Input: part model. Units: mm. Frame: model coordinates. A direction names the side the tool comes from. Coordinates: 2 decimals unless noted, no trailing zeros. Order: outer loops, then holes, each group sorted by start corner. A loop starts at its lowest first (then second) coordinate and runs counter-clockwise, first axis right, second up. Notation, with made-up numbers: M 68.25,22.5 L 80.25,22.5 A14 ccw 80.25,26.5 Z; hole C -31,74.25 d1. An arc over 180 degrees is marked long. Answer in a Markdown table with one row per item.
from build123d import *

# Parameters (mm, degrees)
SKETCH1_W                      = 41.4
SKETCH1_H                      = 33.02
SKETCH1_R                      = 3.175
BOSS_EXTRUDE1_DEPTH            = 12
SKETCH2_W                      = 41.4
SKETCH2_H                      = 6.51
BOSS_EXTRUDE2_DEPTH            = 53
CUT_EXTRUDE1_REACH             = 72.186
SKETCH4_R                      = 3.175
CUT_EXTRUDE1_DIRECTION_2_REACH = 72.186
CUT_EXTRUDE3_REACH             = 72.186
CUT_EXTRUDE3_DIRECTION_2_REACH = 72.186
CUT_EXTRUDE4_DEPTH             = 12
BOSS_EXTRUDE3_DEPTH            = 12
FILLET3_R                      = 3


with BuildPart() as part:
    # Sketch1 → Boss-Extrude1 (new body)
    with BuildSketch(Plane.XY):
        Rectangle(SKETCH1_W, SKETCH1_H)
        with Locations((12.7, 0)):
            Circle(SKETCH1_R, mode=Mode.SUBTRACT)
        with Locations((-12.7, 0)):
            Circle(SKETCH1_R, mode=Mode.SUBTRACT)
    extrude(amount=BOSS_EXTRUDE1_DEPTH)

    # Sketch2 → Boss-Extrude2 (add)
    with BuildSketch(Plane.XY.offset(12)):
        with Locations((0, 13.255)):
            Rectangle(SKETCH2_W, SKETCH2_H)
        with Locations((0, -13.255)):
            Rectangle(SKETCH2_W, SKETCH2_H)
    extrude(amount=BOSS_EXTRUDE2_DEPTH)

    # Cut-Extrude1: up to this face of the body (flat: up to its plane)
    cut_extrude1_end = Plane(part.part.faces().sort_by_distance((0, -16.51, 32.5))[0])
    # Sketch4 → Cut-Extrude1 (cut, up to the picked face)
    with BuildSketch(Plane(origin=(0, 0, 0), x_dir=(1, 0, 0), z_dir=(0, 1, 0)), mode=Mode.PRIVATE) as cut_extrude1_sk1:
        with Locations(Location((0, -35.5, 0), (0, 0, 270))):
            Circle(SKETCH4_R)
    cut_extrude1_tool1 = split(extrude(cut_extrude1_sk1.sketch, amount=-CUT_EXTRUDE1_REACH, mode=Mode.PRIVATE), bisect_by=cut_extrude1_end, keep=Keep.BOTH, mode=Mode.PRIVATE)
    add(cut_extrude1_tool1.solids().sort_by(Axis((0, 0, 35.5), (0, -1, 0)))[0], mode=Mode.SUBTRACT)

    # Cut-Extrude1 direction 2: up to this face of the body (flat: up to its plane)
    cut_extrude1_direction_2_end = Plane(part.part.faces().sort_by_distance((0, 16.51, 32.5))[0])
    # Sketch4 → Cut-Extrude1 direction 2 (cut, up to the picked face)
    with BuildSketch(Plane(origin=(0, 0, 0), x_dir=(1, 0, 0), z_dir=(0, 1, 0)), mode=Mode.PRIVATE) as cut_extrude1_direction_2_sk1:
        with Locations(Location((0, -35.5, 0), (0, 0, 270))):
            Circle(SKETCH4_R)
    cut_extrude1_direction_2_tool1 = split(extrude(cut_extrude1_direction_2_sk1.sketch, amount=CUT_EXTRUDE1_DIRECTION_2_REACH, mode=Mode.PRIVATE), bisect_by=cut_extrude1_direction_2_end, keep=Keep.BOTH, mode=Mode.PRIVATE)
    add(cut_extrude1_direction_2_tool1.solids().sort_by(Axis((0, 0, 35.5), (0, 1, 0)))[0], mode=Mode.SUBTRACT)

    # Cut-Extrude3: up to this face of the body (flat: up to its plane)
    cut_extrude3_end = Plane(part.part.faces().sort_by_distance((-19.929353518, -16.51, 32.5))[0])
    # Sketch6 → Cut-Extrude3 (cut, up to the picked face)
    with BuildSketch(Plane(origin=(0, 0, 0), x_dir=(1, 0, 0), z_dir=(0, 1, 0)), mode=Mode.PRIVATE) as cut_extrude3_sk1:
        with BuildLine():
            Line((-8, -35.5), (-8, -20))
            Line((-8, -20), (-8, -12))
            Line((-8, -12), (-16, -12))
            Line((-16, -12), (-20.7, -12))
            Line((-20.7, -12), (-20.7, -65))
            Line((-20.7, -65), (20.7, -65))
            Line((20.7, -65), (20.7, -12))
            Line((20.7, -12), (16, -12))
            Line((16, -12), (8, -12))
            Line((8, -12), (8, -20))
            Line((8, -20), (8, -35.5))
            ThreePointArc((8, -35.5), (0, -43.5), (-8, -35.5))
        make_face()
    cut_extrude3_tool1 = split(extrude(cut_extrude3_sk1.sketch, amount=-CUT_EXTRUDE3_REACH, mode=Mode.PRIVATE), bisect_by=cut_extrude3_end, keep=Keep.BOTH, mode=Mode.PRIVATE)
    add(cut_extrude3_tool1.solids().sort_by(Axis((-8.67253, 0, 27.75), (0, -1, 0)))[0], mode=Mode.SUBTRACT)

    # Cut-Extrude3 direction 2: up to this face of the body (flat: up to its plane)
    cut_extrude3_direction_2_end = Plane(part.part.faces().sort_by_distance((19.929353518, 16.51, 32.5))[0])
    # Sketch6 → Cut-Extrude3 direction 2 (cut, up to the picked face)
    with BuildSketch(Plane(origin=(0, 0, 0), x_dir=(1, 0, 0), z_dir=(0, 1, 0)), mode=Mode.PRIVATE) as cut_extrude3_direction_2_sk1:
        with BuildLine():
            Line((-8, -35.5), (-8, -20))
            Line((-8, -20), (-8, -12))
            Line((-8, -12), (-16, -12))
            Line((-16, -12), (-20.7, -12))
            Line((-20.7, -12), (-20.7, -65))
            Line((-20.7, -65), (20.7, -65))
            Line((20.7, -65), (20.7, -12))
            Line((20.7, -12), (16, -12))
            Line((16, -12), (8, -12))
            Line((8, -12), (8, -20))
            Line((8, -20), (8, -35.5))
            ThreePointArc((8, -35.5), (0, -43.5), (-8, -35.5))
        make_face()
    cut_extrude3_direction_2_tool1 = split(extrude(cut_extrude3_direction_2_sk1.sketch, amount=CUT_EXTRUDE3_DIRECTION_2_REACH, mode=Mode.PRIVATE), bisect_by=cut_extrude3_direction_2_end, keep=Keep.BOTH, mode=Mode.PRIVATE)
    add(cut_extrude3_direction_2_tool1.solids().sort_by(Axis((-8.67253, 0, 27.75), (0, 1, 0)))[0], mode=Mode.SUBTRACT)

    # Sketch7 → Cut-Extrude4 (cut)
    with BuildSketch(Plane.XY):
        with BuildLine():
            ThreePointArc((-12.7, 7), (-19.7, 0), (-12.7, -7))
            Line((-12.7, -7), (-8, -7))
            Line((-8, -7), (-8, -16.51))
            Line((-8, -16.51), (-20.7, -16.51))
            Line((-20.7, -16.51), (-20.7, 16.51))
            Line((-20.7, 16.51), (-8, 16.51))
            Line((-8, 16.51), (-8, 7))
            Line((-8, 7), (-12.7, 7))
        make_face()
        with BuildLine():
            Line((12.7, 7), (8, 7))
            Line((8, 7), (8, 16.51))
            Line((8, 16.51), (20.7, 16.51))
            Line((20.7, 16.51), (20.7, -16.51))
            Line((20.7, -16.51), (8, -16.51))
            Line((8, -16.51), (8, -7))
            Line((8, -7), (12.7, -7))
            ThreePointArc((12.7, -7), (19.7, 0), (12.7, 7))
        make_face()
    extrude(amount=CUT_EXTRUDE4_DEPTH, mode=Mode.SUBTRACT)

    # Sketch8 → Boss-Extrude3 (add)
    with BuildSketch(Plane.XY):
        with BuildLine():
            Line((8, -16.51), (18.065759147, -4.495400847))
            ThreePointArc((18.065759147, -4.495400847), (15.660759537, -6.343020019), (12.7, -7))
            Line((12.7, -7), (8, -7))
            Line((8, -7), (8, -16.51))
        make_face()
        with BuildLine():
            ThreePointArc((-18.065759147, -4.495400847), (-15.660759537, -6.343020019), (-12.7, -7))
            Line((-12.7, -7), (-8, -7))
            Line((-8, -7), (-8, -16.51))
            Line((-8, -16.51), (-18.065759147, -4.495400847))
        make_face()
        with BuildLine():
            Line((8, 16.51), (18.065759147, 4.495400847))
            ThreePointArc((18.065759147, 4.495400847), (15.660759537, 6.343020019), (12.7, 7))
            Line((12.7, 7), (8, 7))
            Line((8, 7), (8, 16.51))
        make_face()
        with BuildLine():
            Line((-8, 16.51), (-18.065759147, 4.495400847))
            ThreePointArc((-18.065759147, 4.495400847), (-15.660759537, 6.343020019), (-12.7, 7))
            Line((-12.7, 7), (-8, 7))
            Line((-8, 7), (-8, 16.51))
        make_face()
    extrude(amount=BOSS_EXTRUDE3_DEPTH)

    # Fillet3
    fillet3_edges = [part.edges().sort_by_distance(p)[0] for p in [
        (8, -13.255, 12),
        (-8, -13.255, 12),
        (8, 13.255, 12),
        (-8, 13.255, 12),
    ]]
    fillet(fillet3_edges, radius=FILLET3_R)


solid = part.part
1) Reachability of faces 4 (the face through (8, 13, 25)), 5 (the face through (0.95, -13.21, 38.53)), 6 (the face through (-8, -13, 25)) from +Z, -Z, +X, -X, +Y, -Y: full face, straight path, thin tool, end or side. Return the list, or none.
Resolved:
| item | result |
|---|---|
| face 4 | +Z, +X, +Y, -Y |
| face 5 | +Y, -Y |
| face 6 | +Z, -X, +Y, -Y |
2) Cut plane D-D, the plane x = -13. Output: boundary loops of the cut face in (y, z), and give its area (3 significant figures).
Resolved:
| item | result |
|---|---|
| outline | M -10.54,0 L -3.16,0 L -3.16,12 L -10.54,12 Z; M 3.16,0 L 10.54,0 L 10.54,12 L 3.16,12 Z |
| area | 177 mm2 |
3) Cut plane B-B, the plane y = 0. Output: boundary loops of the cut face in (x, z) (3 decimals).
Resolved:
| item | result |
|---|---|
| outline | M -19.7,0 L -15.875,0 L -15.875,12 L -19.7,12 Z; M -9.525,0 L 9.525,0 L 9.525,12 L -9.525,12 Z; M 15.875,0 L 19.7,0 L 19.7,12 L 15.875,12 Z |
4) Cut plane C-C, the plane x = -1.5. Output: boundary loops of the cut face in (y, z), and give its area (3 significant figures).
Resolved:
| item | result |
|---|---|
| outline | M -16.51,0 L 16.51,0 L 16.51,32.7 L 10,32.7 L 10,12 L -10,12 L -10,32.7 L -16.51,32.7 Z; M -16.51,38.3 L -10,38.3 L -10,43.36 L -16.51,43.36 Z; M 10,38.3 L 16.51,38.3 L 16.51,43.36 L 10,43.36 Z |
| area | 732 mm2 |
5) Material intervals for probe 1 along X at (y, z) = (0, 4) (3 decimals); probe 2 along X at (y, z) = (-13, 35.5) (3 decimals); probe 3 along Y at (x, z) = (6.5, 22), sorted ascending.
Resolved:
| item | result |
|---|---|
| probe 1 | x = -19.7 to -15.875, -9.525 to 9.525, 15.875 to 19.7 |
| probe 2 | x = -8 to -3.175, 3.175 to 8 |
| probe 3 | y = -16.51 to -10, 10 to 16.51 |
6) Contact query for flat-ended pins moving along their axis: pin 1 (3.5 mm diameter, centred on y = -12.5, z = 29.5, fed in from +X); pin 2 (3.5 mm diameter, centred on y = -14.5, z = 22, fed in from -X); pin 3 (3 mm diameter, centred on x = 1.5, y = 1, fed in from +Z). Output: stop coordinate, or through.
Resolved:
| item | result |
|---|---|
| pin 1 | stops at x = 8 |
| pin 2 | stops at x = -8 |
| pin 3 | stops at z = 12 |
7) Mould query, pull axis Y, two halves, no side actions, for faces 1 (the face through (0.176, 13.209, 43.498)), 2 (the face through (-9.67, 0.95, 5.92)), 3 (the face through (-12.96, 10.59, 5.73)). Classes: +Y half, -Y half, draft (parallel to the pull), parting line (faces both ways), or undercut.
Resolved:
| item | result |
|---|---|
| face 1 | draft |
| face 2 | undercut |
| face 3 | +Y half |
8) Cut plane A-A, the plane z = 31.5. Output: boundary loops of the cut face in (x, y).
Resolved:
| item | result |
|---|---|
| outline | M -8,-16.51 L 8,-16.51 L 8,-10 L -8,-10 Z; M -8,10 L 8,10 L 8,16.51 L -8,16.51 Z |
